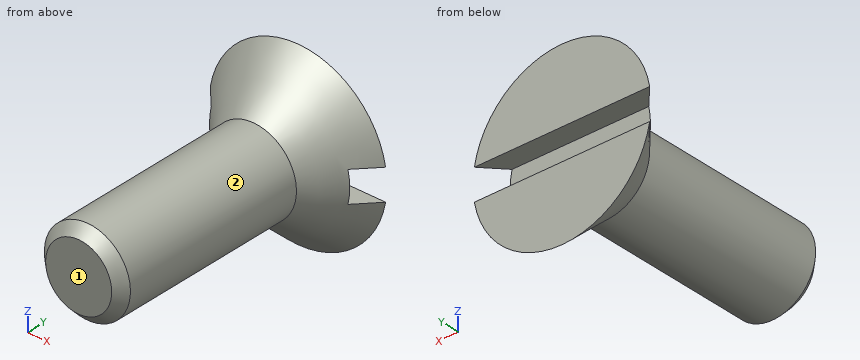
```python
from build123d import *

# Parameters (mm, degrees)
SKETCH1_R     = 1.0922
SHAFT_DEPTH   = 5.08
SKETCH4_W     = 4.517166798
SKETCH4_H     = 0.7874
SLOT_DEPTH    = 0.5334
CHAMFER1_SIZE = 0.254


with BuildPart() as part:
    # Sketch1 → Shaft (new body)
    with BuildSketch(Plane(origin=(0, 0, 0), x_dir=(1, 0, 0), z_dir=(0, 1, 0))):
        with Locations(Location((0, 0, 0), (0, 0, 270))):
            Circle(SKETCH1_R)
    extrude(amount=-SHAFT_DEPTH)

    # Sketch3 → Head (revolve)
    with BuildSketch(Plane.XY, mode=Mode.PRIVATE) as head_sk:
        Polygon((0, 0), (0, 1.2954), (2.258583399, 1.2954), (1.0922, 0), align=None)
    revolve(head_sk.sketch.rotate(Axis((0, 0, 0), (0, 1, 0)), 270), axis=Axis((0, 0, 0), (0, 1, 0)))

    # Sketch4 → Slot (cut)
    with BuildSketch(Plane(origin=(0, 1.2954, 0), x_dir=(1, 0, 0), z_dir=(0, 1, 0))):
        Rectangle(SKETCH4_W, SKETCH4_H)
    extrude(amount=-SLOT_DEPTH, mode=Mode.SUBTRACT)

    # Chamfer1
    chamfer1_edges = [part.edges().sort_by_distance(p)[0] for p in [
        (0, -5.08, -1.0922),
    ]]
    chamfer(chamfer1_edges, length=CHAMFER1_SIZE)


solid = part.part
```
Read the model definition and answer for the solid it produces. Units are mm, in the model's axes. Face numbers are marked on the shaded views. A direction names the side the tool comes from. Round coordinates to 2 decimals unless told otherwise and drop trailing zeros. Write each loop counter-clockwise with the first axis right and the second up, starting at its lowest first coordinate (ties: lowest second). Pieces come first, ordered by that corner, then holes. Notation, with made-up numbers: (5, -5) -> (28, -5) arc R33 cw to (28, 33) -> close; hole circle Ø2 at (4, -21). An arc over 180 degrees is marked (long way). Answer in a Markdown table with one row per item. Add a question column.
1) Given P1, Ø2, axis at x = 1, y = -0.5, coming from the +Z side, flat-ended and moving along its own axis, determine where the tip first touches the part or whether it passes through.
2) Find section B-B, the plane z = 0. Determine the outline of the cut face in (x, y).
3) Find section C-C, the plane y = -3. Determine the outline of the cut face in (x, z).
4) Find section A-A, the plane x = 0. Determine the outline of the cut face in (y, z).
5) Which of the six approach directions +Z, -Z, +X, -X, +Y, -Y give full straight-line access (tool end or side, diameter ignored) to the marked faces 1 and 2?
6) Consider line 1 (X direction, y = -0.25, z = 0.05); line 2 (Y direction, x = 0.3, z = -0.2); line 3 (Z direction, x = -1.05, y = 1). Determine where each line is inside the solid, lowest interval first.
Findings below:
| question | item | result |
|---|---|---|
| 1 | P1 | z = 1.34 |
| 2 | outline | (-1.78, 0.76) -> (-1.09, 0) -> (-1.09, -4.83) -> (-0.84, -5.08) -> (0.84, -5.08) -> (1.09, -4.83) -> (1.09, 0) -> (1.78, 0.76) -> close |
| 3 | outline | circle Ø2.18 at (0, 0) |
| 4 | outline | (-5.08, -0.84) -> (-4.83, -1.09) -> (0, -1.09) -> (1.3, -2.26) -> (1.3, -0.39) -> (0.76, -0.39) -> (0.76, 0.39) -> (1.3, 0.39) -> (1.3, 2.26) -> (0, 1.09) -> (-4.83, 1.09) -> (-5.08, 0.84) -> close |
| 5 | face 1 | +Z, -Z, +X, -X, -Y |
| 5 | face 2 | -Y |
| 6 | line 1 | -1.09 to 1.09 |
| 6 | line 2 | -5.08 to 0.76 |
| 6 | line 3 | -1.69 to -0.39, 0.39 to 1.69 |
